Build history of the part. All positions in model axes, mm. A direction names the side the tool comes from. Give positions to 0.01 mm unless a question says otherwise; leave off trailing zeros. Write each loop counter-clockwise with the first axis right and the second up, starting at its lowest first coordinate (ties: lowest second). Pieces come first, ordered by that corner, then holes. Notation, with made-up numbers: (25.25, 8) -> (80.25, 8) arc R11 ccw to (80.25, 26) -> close; hole circle Ø7 at (43, -25). An arc over 180 degrees is marked (long way). Put each result on its own line as item: value. Start each with the question number.
Item 1: Slice it at C-C, the plane y = -7.25. List the corners of the cut face in (x, z).
Item 2: Drill centre lines: line 1 along Y through (x, z) = (1.35, 1.05); line 2 along Y through (x, z) = (0.55, 0.8); line 3 along X through (y, z) = (-10, -0.65). Where is each one in solid material? Low to high.
Item 3: Slice it at A-A, the plane z = 0. List the corners of the cut face in (x, y), plus the area to 3 significant figures.
Item 4: Tool access for faces 1 (the cylindrical face through (0, -6, 1)), 2 (the flat face through (0, 2, 0)): list every direction of +Z, -Z, +X, -X, +Y, -Y with a clear straight run to the whole face (end or side of a thin tool).
Item 5: Flat gauge pin, fed straight in: pin 1 Ø1 at (y, z) = (-6, 0.5) entering from -X. Where does the tip first touch, or does it go through?
Item 6: Slice it at B-B, the plane x = 0. List the corners of the cut face in (y, z).
```python
from build123d import *

# Parameters (mm, degrees)
SKETCH1_W           = 3.5
SKETCH1_H           = 3.5
BOSS_EXTRUDE1_DEPTH = 2
SKETCH2_R           = 1
BOSS_EXTRUDE2_DEPTH = 12
CHAMFER1_SIZE       = 0.3


with BuildPart() as part:
    # Sketch1 → Boss-Extrude1 (new body)
    with BuildSketch(Plane(origin=(0, 0, 0), x_dir=(1, 0, 0), z_dir=(0, 1, 0))):
        Rectangle(SKETCH1_W, SKETCH1_H)
    extrude(amount=BOSS_EXTRUDE1_DEPTH)

    # Sketch2 → Boss-Extrude2 (add)
    with BuildSketch(Plane(origin=(0, 0, 0), x_dir=(1, 0, 0), z_dir=(0, 1, 0))):
        Circle(SKETCH2_R)
    extrude(amount=-BOSS_EXTRUDE2_DEPTH)

    # Chamfer1
    chamfer1_edges = [part.edges().sort_by_distance(p)[0] for p in [
        (-1, -12, 0),
        (-1.75, 1, -1.75),
        (1.75, 1, -1.75),
        (1.75, 1, 1.75),
        (-1.75, 1, 1.75),
    ]]
    chamfer(chamfer1_edges, length=CHAMFER1_SIZE)


solid = part.part
```
Values follow:
1. outline: circle Ø2 at (0, 0)
2. line 1: 0 to 2
2. line 2: -11.73 to 2
2. line 3: -0.76 to 0.76
3. outline: (-1.75, 0) -> (-1, 0) -> (-1, -11.7) -> (-0.7, -12) -> (0.7, -12) -> (1, -11.7) -> (1, 0) -> (1.75, 0) -> (1.75, 2) -> (-1.75, 2) -> close
3. area: 30.9 mm2
4. face 1: -Y
4. face 2: +Z, -Z, +X, -X, +Y
5. pin 1: x = -1
6. outline: (-12, -0.7) -> (-11.7, -1) -> (0, -1) -> (0, -1.75) -> (2, -1.75) -> (2, 1.75) -> (0, 1.75) -> (0, 1) -> (-11.7, 1) -> (-12, 0.7) -> close
